For this review, take the finished solid that the model builds, in its own axes (mm). Face numbers are marked on the shaded views. A direction names the side the tool comes from. Round coordinates to 2 decimals unless told otherwise and drop trailing zeros. Write each loop counter-clockwise with the first axis right and the second up, starting at its lowest first coordinate (ties: lowest second). Pieces come first, ordered by that corner, then holes. Notation, with made-up numbers: (75, 50.25) -> (83, 50.25) arc R34 cw to (83, 82.25) -> close; hole circle Ø10 at (-1, 37). An arc over 180 degrees is marked (long way). Answer as CSV lines item,"result". Start each with the question number.
Item 1: Machinability: for the marked faces 1, 2, 3, 4 and 5, which of the approach directions +Z, -Z, +X, -X, +Y, -Y give a long, thin tool a straight path to every point of the face, cutting with its end or side? Answer none if there is none.
Item 2: Wall thickness on probe 1 along X at (y, z) = (45, 2.75); probe 2 along Y at (x, z) = (74.5, 2.8); probe 3 along Y at (x, z) = (10.5, 27.5): over which ranges is each line inside the solid? List them lowest first. Write a range as from..to.
Item 3: Take a section at D-D on y = 29. Give the boundary of the cut face in (x, z), then the cut area to 3 significant figures.
Item 4: Take a section at B-B on x = 10.5. Give the boundary of the cut face in (y, z).
Item 5: Take a section at C-C on y = 45. Give the boundary of the cut face in (x, z), then the cut area to 3 significant figures.
Item 6: For pin 1 Ø5 at (x, y) = (16, 16) entering from -Z; pin 2 Ø4.5 at (x, y) = (10.5, 45) entering from +Z; pin 3 Ø13 at (x, y) = (93, 51) entering from +Z; pin 4 Ø4 at (x, z) = (95, 7.5) entering from -Y, all flat-tipped, find the tip position at first contact; note any pin that passes through.
Item 7: Take a section at A-A on z = 18.5. Give the boundary of the cut face in (x, y).
```python
from build123d import *

# Parameters (mm, degrees)
SKETCH_1_W          = 85
SKETCH_1_H          = 58
SKETCH_1_R          = 1.75
EXTRUDE_1_DEPTH     = 36
SKETCH_2_R          = 3
CUT_EXTRUDE_1_DEPTH = 31
SKETCH_5_W          = 8
SKETCH_5_H          = 16
EXTRUDE_867_DEPTH   = 16
SKETCH_6_W          = 10
SKETCH_6_H          = 20
EXTRUDE_2_DEPTH     = 16
CHAMFER_1_SIZE      = 10


with BuildPart() as part:
    # 草图1 → 凸台-拉伸1 (new body)
    with BuildSketch(Plane.XY):
        with Locations((42.5, 29)):
            Rectangle(SKETCH_1_W, SKETCH_1_H)
        with Locations((10.5, 45)):
            Circle(SKETCH_1_R, mode=Mode.SUBTRACT)
        with Locations((74.5, 45)):
            Circle(SKETCH_1_R, mode=Mode.SUBTRACT)
        with Locations((10.5, 13)):
            Circle(SKETCH_1_R, mode=Mode.SUBTRACT)
        with Locations((74.5, 13)):
            Circle(SKETCH_1_R, mode=Mode.SUBTRACT)
    extrude(amount=EXTRUDE_1_DEPTH)

    # 草图2 → 切除-拉伸1 (cut)
    with BuildSketch(Plane.XY.offset(36)):
        with Locations((10.5, 45)):
            Circle(SKETCH_2_R)
        with Locations((74.5, 45)):
            Circle(SKETCH_2_R)
        with Locations((74.5, 13)):
            Circle(SKETCH_2_R)
        with Locations((10.5, 13)):
            Circle(SKETCH_2_R)
    extrude(amount=-CUT_EXTRUDE_1_DEPTH, mode=Mode.SUBTRACT)

    # 草图5 → Extrude 867 (add)
    with BuildSketch(Plane(origin=(85, 0, 0), x_dir=(0, 0, -1), z_dir=(1, 0, 0))):
        with Locations((-6, 29)):
            Rectangle(SKETCH_5_W, SKETCH_5_H)
    extrude(amount=EXTRUDE_867_DEPTH)

    # 草图6 → 凸台-拉伸2 (add)
    with BuildSketch(Plane(origin=(85, 0, 0), x_dir=(0, 0, -1), z_dir=(1, 0, 0))):
        with Locations((-17, 48)):
            Rectangle(SKETCH_6_W, SKETCH_6_H)
        with Locations((-17, 10)):
            Rectangle(SKETCH_6_W, SKETCH_6_H)
    extrude(amount=EXTRUDE_2_DEPTH)

    # 倒角1
    chamfer_1_edges = [part.edges().sort_by_distance(p)[0] for p in [
        (101, 58, 17),
        (101, 0, 17),
    ]]
    chamfer(chamfer_1_edges, length=CHAMFER_1_SIZE)


solid = part.part
```
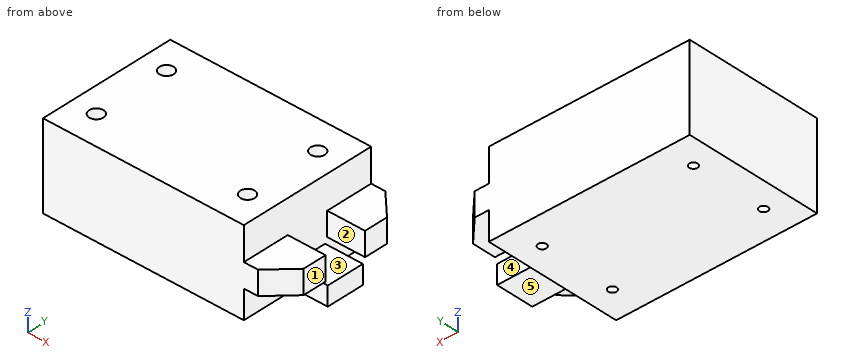
Output values:
1,face 1,"+Z, -Z, +X, +Y, -Y"
1,face 2,"+Z, -Z, +X"
1,face 3,"+Z, +X, +Y, -Y"
1,face 4,"+Z, -Z, +X, +Y"
1,face 5,"-Z, +X, +Y, -Y"
2,probe 1,"x = 0..8.75, 12.25..72.75, 76.25..85"
2,probe 2,"y = 0..11.25, 14.75..43.25, 46.75..58"
2,probe 3,"y = 0..10, 16..42, 48..58"
3,outline,"(0, 0) -> (85, 0) -> (85, 2) -> (101, 2) -> (101, 10) -> (85, 10) -> (85, 36) -> (0, 36) -> close"
3,area,"3,190 mm^2"
4,outline,"(0, 0) -> (11.25, 0) -> (11.25, 5) -> (10, 5) -> (10, 36) -> (0, 36) -> close; (14.75, 0) -> (43.25, 0) -> (43.25, 5) -> (42, 5) -> (42, 36) -> (16, 36) -> (16, 5) -> (14.75, 5) -> close; (46.75, 0) -> (58, 0) -> (58, 36) -> (48, 36) -> (48, 5) -> (46.75, 5) -> close"
5,outline,"(0, 0) -> (8.75, 0) -> (8.75, 5) -> (7.5, 5) -> (7.5, 36) -> (0, 36) -> close; (12.25, 0) -> (72.75, 0) -> (72.75, 5) -> (71.5, 5) -> (71.5, 36) -> (13.5, 36) -> (13.5, 5) -> (12.25, 5) -> close; (76.25, 0) -> (85, 0) -> (85, 12) -> (101, 12) -> (101, 22) -> (85, 22) -> (85, 36) -> (77.5, 36) -> (77.5, 5) -> (76.25, 5) -> close"
5,area,"2,810 mm^2"
6,pin 1,"stops at z = 0"
6,pin 2,"stops at z = 5"
6,pin 3,"stops at z = 22"
6,pin 4,"stops at y = 21"
7,outline,"(0, 0) -> (91, 0) -> (101, 10) -> (101, 20) -> (85, 20) -> (85, 38) -> (101, 38) -> (101, 48) -> (91, 58) -> (0, 58) -> close; hole circle Ø6 at (10.5, 13); hole circle Ø6 at (10.5, 45); hole circle Ø6 at (74.5, 13); hole circle Ø6 at (74.5, 45)"
